Can you work these out from the model? Positions are in its coordinate system, mm. A direction names the side the tool comes from. Give positions to 0.01 mm unless a question says otherwise; leave off trailing zeros. Write each loop counter-clockwise with the first axis right and the second up, starting at its lowest first coordinate (ties: lowest second). Pieces come first, ordered by that corner, then holes.
from build123d import *

# Parameters (mm, degrees)
F0_R     = 17.145
F1_DEPTH = 50.8


# Not quite as in the source:
# - a feature names something its author has since deleted; it is built from what else it names


with BuildPart() as f1:
    # F0 (on Front) → F1 (new body)
    with BuildSketch(Plane.XZ):
        with BuildLine():
            Line((4.6743845872, 28.1900825421), (0, 28.575))
            ThreePointArc((0, 28.575), (-28.575, 0), (0, -28.575))
            Line((0, -28.575), (4.6743845872, -28.1900825421))
            ThreePointArc((4.6743845872, -28.1900825421), (21.7956551241, -18.4791786265), (28.575, 0))
            ThreePointArc((28.575, 0), (21.7956551241, 18.4791786265), (4.6743845872, 28.1900825421))
        make_face()
        with BuildLine():
            ThreePointArc((-13.7262649311, -10.27329918), (-17.145, 0), (-13.7262649311, 10.27329918))
            ThreePointArc((-13.7262649311, 10.27329918), (0, 17.145), (13.7262649311, 10.27329918))
            Line((13.7262649311, 10.27329918), (22.7799285203, 10.27329918))
            Line((22.7799285203, 10.27329918), (22.7799285203, -10.27329918))
            Line((22.7799285203, -10.27329918), (13.7262649311, -10.27329918))
            ThreePointArc((13.7262649311, -10.27329918), (0, -17.145), (-13.7262649311, -10.27329918))
        make_face(mode=Mode.SUBTRACT)
        with BuildLine():
            ThreePointArc((4.6743845872, 28.1900825421), (2.3451030211, 28.4786080562), (0, 28.575))
            Line((0, 28.575), (4.6743845872, 28.1900825421))
        make_face()
        with BuildLine():
            Line((4.6743845872, -28.1900825421), (0, -28.575))
            ThreePointArc((0, -28.575), (2.3451030211, -28.4786080562), (4.6743845872, -28.1900825421))
        make_face()
        with BuildLine():
            Line((78.0239690164, 22.1500284882), (4.6743845872, 28.1900825421))
            ThreePointArc((4.6743845872, 28.1900825421), (21.7956551241, 18.4791786265), (28.575, 0))
            ThreePointArc((28.575, 0), (21.7956551241, -18.4791786265), (4.6743845872, -28.1900825421))
            Line((4.6743845872, -28.1900825421), (78.0239690164, -22.1500284882))
            ThreePointArc((78.0239690164, -22.1500284882), (53.975, 0), (78.0239690164, 22.1500284882))
        make_face()
        with BuildLine():
            ThreePointArc((98.425, 0), (92.5476043564, 15.0567744489), (78.0239690164, 22.1500284882))
            ThreePointArc((78.0239690164, 22.1500284882), (53.975, 0), (78.0239690164, -22.1500284882))
            ThreePointArc((78.0239690164, -22.1500284882), (92.5476043564, -15.0567744489), (98.425, 0))
        make_face()
        with Locations((76.2, 0)):
            Circle(F0_R, mode=Mode.SUBTRACT)
    extrude(amount=F1_DEPTH)


solid = f1.part
(1) Imagine slicing it at C-C, the plane z = -8. Write out the boundary of the cut face in (x, y), plus the area to 3 significant figures.
Returned:
outline: (-27.43, -50.8) - (-15.16, -50.8) - (-15.16, 0) - (-27.43, 0) - close; (22.78, -50.8) - (61.04, -50.8) - (61.04, 0) - (22.78, 0) - close; (91.36, -50.8) - (96.94, -50.8) - (96.94, 0) - (91.36, 0) - close
area: 2,850 mm2
(2) For faces 5 (the face through (22.78, -25, 0)), 6 (the face through (40.84, -25.04, -25.21)), which set-ups out of +Z, -Z, +X, -X, +Y, -Y let a thin tool reach every point of the face, with its end or its side?
Returned:
face 5: +Y, -Y
face 6: -Z, +X, +Y, -Y
(3) Imagine slicing it at D-D, the plane x = 70.5. Write out the boundary of the cut face in (y, z), plus the area to 3 significant figures.
Returned:
outline: (-50.8, -22.77) - (0, -22.77) - (0, -16.17) - (-50.8, -16.17) - close; (-50.8, 16.17) - (0, 16.17) - (0, 22.77) - (-50.8, 22.77) - close
area: 671 mm2
(4) If we mould it in two halves opening along Z, with no side actions, what happens to faces 1 (the face through (63.563, -25.044, 11.587)), 2 (the face through (18, -25, -10.273)), 3 (the face through (34, 0, 0)), 4 (the face through (41.863, -25.044, 25.128))? For each: +Z half, -Z half, draft (parallel to the pull), parting line (faces both ways), or undercut.
Returned:
face 1: undercut
face 2: undercut
face 3: draft
face 4: +Z half
(5) Will these pins go through, and if not, where does the flat tip stop? P1, Ø5, axis at y = -15, z = 14, coming from the +X side; P2, Ø5, axis at y = -6.5, z = 11.5, coming from the +X side; P3, Ø5, axis at x = -6, y = -19.5, coming from the +Z side; P4, Ø6, axis at x = -5.5, z = 10, coming from the -Y side.
Returned:
P1: stops at x = 95.22
P2: stops at x = 96.52
P3: stops at z = 28.36
P4: passes through
(6) Imagine slicing it at B-B, the plane x = -7. Write out the boundary of the cut face in (y, z), plus the area to 3 significant figures.
Returned:
outline: (-50.8, -27.7) - (0, -27.7) - (0, -15.65) - (-50.8, -15.65) - close; (-50.8, 15.65) - (0, 15.65) - (0, 27.7) - (-50.8, 27.7) - close
area: 1,220 mm2
(7) Imagine slicing it at A-A, the plane y = -42. Write out the boundary of the cut face in (x, z) (3 decimals).
Returned:
outline: (4.674, -28.19) - (78.024, -22.15) arc R22.225 ccw to (78.024, 22.15) - (4.674, 28.19) arc R28.575 ccw (long way) to start; hole (13.726, -10.273) - (22.78, -10.273) - (22.78, 10.273) - (13.726, 10.273) arc R17.145 ccw (long way) to start; hole circle Ø34.29 at (76.2, 0)
(8) If I drill on L1, parallel to X at y = -38, z = -7; L2, parallel to X at y = -30, z = 11.5; L3, parallel to Z at x = 18.5, y = -18.5, over which ranges is the centre line in solid material (lowest first)?
Returned:
L1: x = -27.7 to -15.65, 22.78 to 60.55, 91.85 to 97.29
L2: x = -26.16 to -12.72, 12.72 to 63.48, 88.92 to 95.22
L3: z = -27.05 to -10.27, 10.27 to 27.05
